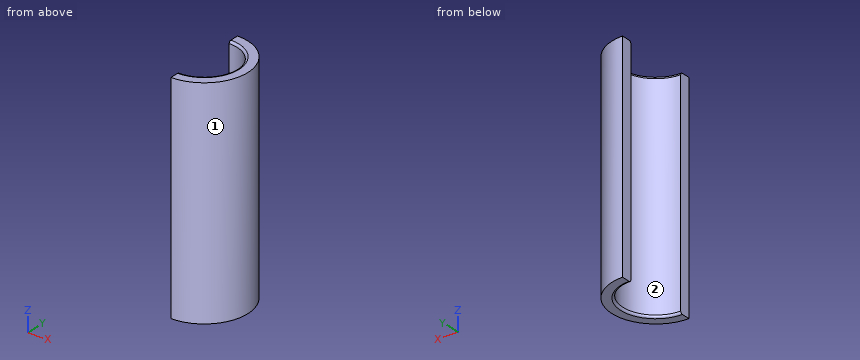
from build123d import *

# Parameters (mm, degrees)
AUFSATZ_LINEAR_AUSTRAGEN1_DEPTH = 100
VERRUNDUNG1_R                   = 2


with BuildPart() as part:
    # Skizze1 → Aufsatz-Linear austragen1 (new, symmetric)
    with BuildSketch(Plane.XY):
        with BuildLine():
            Line((0, 40), (0, 30))
            ThreePointArc((0, 30), (30, 0), (0, -30))
            Line((0, -30), (0, -40))
            ThreePointArc((0, -40), (40, 0), (0, 40))
        make_face()
    extrude(amount=AUFSATZ_LINEAR_AUSTRAGEN1_DEPTH, both=True)

    # Verrundung1
    verrundung1_edges = [part.edges().sort_by_distance(p)[0] for p in [
        (30, 0, 100),
        (30, 0, -100),
    ]]
    fillet(verrundung1_edges, radius=VERRUNDUNG1_R)


solid = part.part
Design review of the part built by this model. Coordinates are the model's own, in mm. Face numbers are marked on the shaded views. Coordinates: 2 decimals unless noted, no trailing zeros. Order: outer loops, then holes, each group sorted by start corner. A loop starts at its lowest first (then second) coordinate and runs counter-clockwise, first axis right, second up.
Item 1: The part is to be moulded in two halves that separate along Y. For the marked faces 1 and 2, say which applies: pulls with the +Y half, pulls with the -Y half, needs draft (parallel to the pull), parting line crosses it, or undercut.
Item 2: Take a section at B-B, the plane z = -56. Write out the cut boundary in (x, y), then the cut area to 3 significant figures.
Item 3: For pin 1 Ø2 at (x, z) = (4.5, 25) entering from +Y; pin 2 Ø10 at (y, z) = (-12.5, 6) entering from -X; pin 3 Ø1 at (x, z) = (21.5, 11.5) entering from -Y, all flat-tipped, find the tip position at first contact; note any pin that passes through.
Item 4: For line 1 (Y direction, x = 24, z = -71); line 2 (Y direction, x = 3, z = 6); line 3 (X direction, y = 31, z = -61), list the stretches that pass through material, from the lowest coordinate up.
Item 5: Take a section at A-A, the plane y = 0. Write out the cut boundary in (x, z).
Item 6: Take a section at C-C, the plane y = -34.5. Write out the cut boundary in (x, z).
The answers:
1. face 1: parting line crosses it
1. face 2: undercut
2. outline: (0, -40) arc R40 ccw to (0, 40) - (0, 30) arc R30 cw to (0, -30) - close
2. area: 1,100 mm2
3. pin 1: stops at y = 39.85
3. pin 2: stops at x = 24.37
3. pin 3: stops at y = -34.04
4. line 1: y = -32 to -18, 18 to 32
4. line 2: y = -39.89 to -29.85, 29.85 to 39.89
4. line 3: x = 0 to 25.28
5. outline: (30, -98) arc R2 ccw to (32, -100) - (40, -100) - (40, 100) - (32, 100) arc R2 ccw to (30, 98) - close
6. outline: (0, -100) - (20.24, -100) - (20.24, 100) - (0, 100) - close
